from build123d import *

# Parameters (mm, degrees)
ESQUISSE1_W                  = 18
ESQUISSE1_H                  = 7.75
BOSS_EXTRU_1_DEPTH           = 5
ENL_V_MAT_EXTRU_1_DEPTH      = 15
ENL_V_MAT_EXTRU_1_DEPTH_BACK = 10
ESQUISSE13_RX                = 0.8
ESQUISSE13_RY                = 0.6
ESQUISSE15_R                 = 0.25
BOSS_EXTRU_3_DEPTH           = 0.5


with BuildPart() as part:
    # Esquisse1 → Boss.-Extru.1 (new body)
    with BuildSketch(Plane.XY):
        with Locations((9, 3.875)):
            Rectangle(ESQUISSE1_W, ESQUISSE1_H)
    extrude(amount=BOSS_EXTRU_1_DEPTH)

    # Esquisse13 → Enl_v. mat.-Extru.1 (cut, two sides: drawn at the far end of the back side and taken through both)
    with BuildSketch(Plane(origin=(5, 3.875, 5), x_dir=(-0.7071067811865476, 0, -0.7071067811865475), z_dir=(0.7071067811865475, 0, -0.7071067811865476)).offset(-ENL_V_MAT_EXTRU_1_DEPTH_BACK)):
        with Locations(Location((0, 0), (0, 0, 0))):
            Ellipse(ESQUISSE13_RX, ESQUISSE13_RY)
    extrude(amount=ENL_V_MAT_EXTRU_1_DEPTH + ENL_V_MAT_EXTRU_1_DEPTH_BACK, mode=Mode.SUBTRACT)

    # Esquisse15 → Boss.-Extru.3 (add)
    with BuildSketch(Plane(origin=(0, 0, 0), x_dir=(-1, 0, 0), z_dir=(0, 0, -1))):
        with Locations(Location((-11.729236125, 2.125, 0), (0, 0, 180))):
            Circle(ESQUISSE15_R)
        with Locations(Location((-11.729236125, 5.625, 0), (0, 0, 180))):
            Circle(ESQUISSE15_R)
    extrude(amount=BOSS_EXTRU_3_DEPTH)


solid = part.part
Input: part model. Units: mm. Frame: model coordinates. Give positions to 0.01 mm unless a question says otherwise; leave off trailing zeros. Write each loop counter-clockwise with the first axis right and the second up, starting at its lowest first coordinate (ties: lowest second). Pieces come first, ordered by that corner, then holes. Notation, with made-up numbers: M 5.25,58 L 16.25,58 A23 ccw 16.25,70 Z; hole C 74.25,39 d3. An arc over 180 degrees is marked long. Use one line per item in the form item = value.
1. First-contact query: P1, Ø1, axis at x = 11.5, y = 3.5, coming from the -Z side. Flat tip, straight axial feed; report the tip coordinate or a pass-through.
Outcome:
P1 = 0
2. Ray query, L1, parallel to Z at x = 1.25, y = 5.75; L2, parallel to Y at x = 6, z = 2.95; L3, parallel to Y at x = 8.5, z = 1.7. Return the intervals inside material, ascending.
Outcome:
L1 = 0 to 5
L2 = 0 to 3.65, 4.1 to 7.75
L3 = 0 to 3.28, 4.47 to 7.75
3. Cut plane B-B on y = 6.5. Return loops of the section in (x, z), and give its area (3 significant figures).
Outcome:
outline = M 0,0 L 18,0 L 18,5 L 0,5 Z
area = 90.0 mm²
4. Cut plane A-A on x = 11.75. Return loops of the section in (y, z).
Outcome:
outline = M 0,0 L 1.88,0 L 1.88,-0.5 L 2.37,-0.5 L 2.37,0 L 5.38,0 L 5.38,-0.5 L 5.87,-0.5 L 5.87,0 L 7.75,0 L 7.75,5 L 0,5 Z
